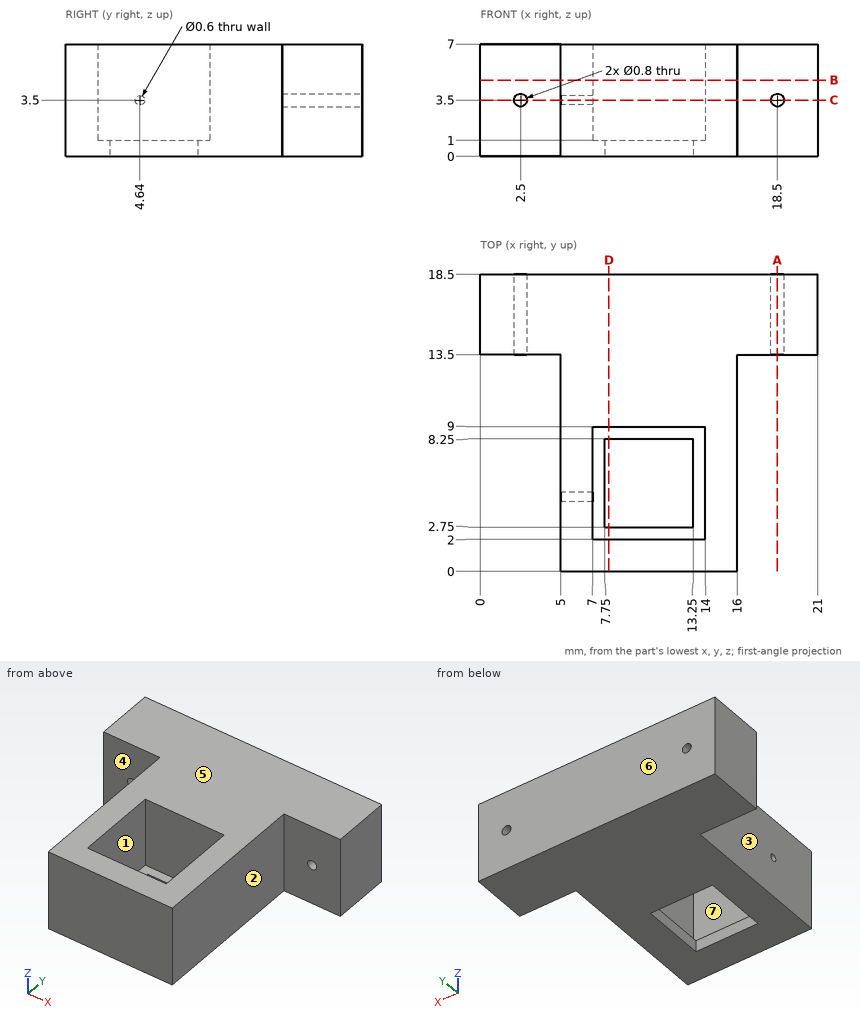
Could you check a few things on this drawing? It's one solid part, dimensions in mm from its lowest x, y, z. A direction names the side the tool comes from. Give positions to 0.01 mm unless a question says otherwise; leave off trailing zeros. Order: outer loops, then holes, each group sorted by start corner. A loop starts at its lowest first (then second) coordinate and runs counter-clockwise, first axis right, second up. Notation, with made-up numbers: M 23,40.25 L 28,40.25 A22 cw 28,76.25 Z; hole C 70.5,68 d10. An arc over 180 degrees is marked long. Use one line per item in the form item = value. Start each with the question number.
Item 1: If we section it at B-B (z = 4.75): Write out the boundary of the cut face in (x, y), then the cut area to 4 significant figures.
Item 2: If we section it at C-C (z = 3.5): Write out the boundary of the cut face in (x, y).
Item 3: For the marked faces 1, 2 and 3, which set-ups out of +Z, -Z, +X, -X, +Y, -Y let a thin tool reach every point of the face, with its end or its side?
Item 4: If we section it at A-A (x = 18.5): Write out the boundary of the cut face in (y, z).
Item 5: If I drill on line 1 along X through (y, z) = (14.75, 3.5); line 2 along Y through (x, z) = (5.65, 3.5); line 3 along Y through (x, z) = (13.25, 5.75), over which ranges is the centre line in solid material (lowest first)?
Item 6: Will these pins go through, and if not, where does the flat tip stop? pin 1 Ø2.5 at (x, z) = (18, 2.5) entering from -Y; pin 2 Ø2 at (y, z) = (7.5, 4.5) entering from -X; pin 3 Ø1.5 at (y, z) = (12, 2.5) entering from +X.
Item 7: If we section it at D-D (x = 8): Write out the boundary of the cut face in (y, z), then the cut area to 3 significant figures.
Item 8: We'd pull the mould along Y, two halves only. Please class the marked faces 4, 5, 6 and 7: +Y half, -Y half, draft (parallel to the pull), parting line (faces both ways), or undercut.
Outcome:
q1.outline = M 0,13.5 L 5,13.5 L 5,0 L 16,0 L 16,13.5 L 21,13.5 L 21,18.5 L 0,18.5 Z; hole M 7,2 L 14,2 L 14,9 L 7,9 Z
q1.area = 204.5 mm2
q2.outline = M 0,13.5 L 2.1,13.5 L 2.1,18.5 L 0,18.5 Z; M 2.9,13.5 L 5,13.5 L 5,4.94 L 7,4.94 L 7,9 L 14,9 L 14,2 L 7,2 L 7,4.34 L 5,4.34 L 5,0 L 16,0 L 16,13.5 L 18.1,13.5 L 18.1,18.5 L 2.9,18.5 Z; M 18.9,13.5 L 21,13.5 L 21,18.5 L 18.9,18.5 Z
q3.face_1 = +Z
q3.face_2 = +Z, -Z, +X, -Y
q3.face_3 = +Z, -Z, -X, -Y
q4.outline = M 13.5,0 L 18.5,0 L 18.5,3.1 L 13.5,3.1 Z; M 13.5,3.9 L 18.5,3.9 L 18.5,7 L 13.5,7 Z
q5.line_1 = 0 to 2.1, 2.9 to 18.1, 18.9 to 21
q5.line_2 = 0 to 4.34, 4.94 to 18.5
q5.line_3 = 0 to 2, 9 to 18.5
q6.pin_1 = 13.5
q6.pin_2 = 5
q6.pin_3 = 16
q7.outline = M 0,0 L 2.75,0 L 2.75,1 L 2,1 L 2,7 L 0,7 Z; M 8.25,0 L 18.5,0 L 18.5,7 L 9,7 L 9,1 L 8.25,1 Z
q7.area = 82.0 mm2
q8.face_4 = -Y half
q8.face_5 = draft
q8.face_6 = +Y half
q8.face_7 = undercut
